Drawing for the job (mm, zero at the part's lowest x, y, z). A direction names the side the tool comes from. Give positions to 0.01 mm unless a question says otherwise; leave off trailing zeros. Order: outer loops, then holes, each group sorted by start corner. A loop starts at its lowest first (then second) coordinate and runs counter-clockwise, first axis right, second up. Notation, with made-up numbers: (23, 0) - (31, 0) arc R11 ccw to (31, 19) - close; hole circle Ø9 at (8, 51.5). An arc over 180 degrees is marked (long way). Use a Markdown table: item, result.
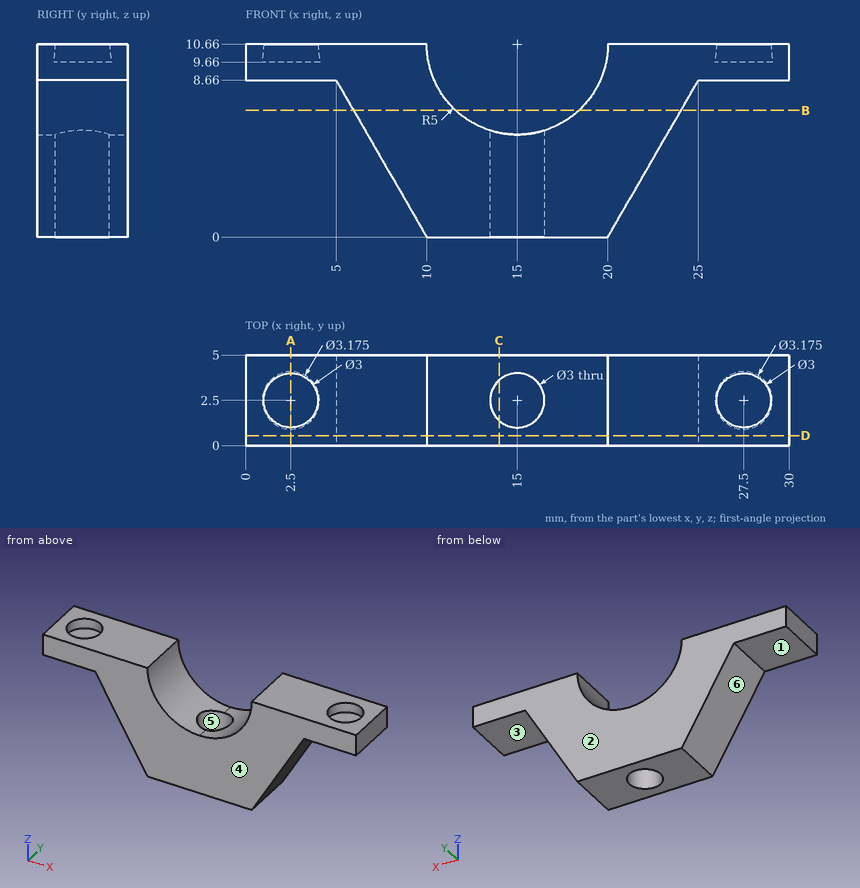
1) Two-plate mould, pull along X, no slides. Class the marked faces 4, 5 and 6: +X half, -X half, draft (parallel to the pull), parting line (faces both ways), or undercut.
Computed:
| item | result |
|---|---|
| face 4 | draft |
| face 5 | undercut |
| face 6 | -X half |
2) Slice it at D-D (y = 0.55). Write the cut outline in (x, z).
Computed:
| item | result |
|---|---|
| outline | (0, 8.66) - (5, 8.66) - (10, 0) - (20, 0) - (25, 8.66) - (30, 8.66) - (30, 10.66) - (20, 10.66) arc R5 cw to (10, 10.66) - (0, 10.66) - close |
3) Wall check: line 1 (Y direction, x = 15, z = 1.8); line 2 (Z direction, x = 27, y = 4.2); line 3 (X direction, y = 2.7, z = 5.75). Give the ranges that are in metal, low to high. Write a range as from..to.
Computed:
| item | result |
|---|---|
| line 1 | y = 0..1, 4..5 |
| line 2 | z = 8.66..10.66 |
| line 3 | x = 6.68..13.51, 16.49..23.32 |
4) Tool access for the marked faces 1, 2 and 3: list every direction of +Z, -Z, +X, -X, +Y, -Y with a clear straight run to the whole face (end or side of a thin tool).
Computed:
| item | result |
|---|---|
| face 1 | -Z, -X, +Y, -Y |
| face 2 | +Z, -Z, +X, -X, +Y |
| face 3 | -Z, +X, +Y, -Y |
5) Pin check, flat tip, straight feed: P1, Ø1.8, axis at x = 15, y = 2.5, coming from the +Z side. Stop position of the tip, or through.
Computed:
| item | result |
|---|---|
| P1 | passes through |
6) Slice it at B-B (z = 7). Write the cut outline in (x, y).
Computed:
| item | result |
|---|---|
| outline | (5.96, 0) - (11.59, 0) - (11.59, 5) - (5.96, 5) - close; (18.41, 0) - (24.04, 0) - (24.04, 5) - (18.41, 5) - close |
7) Slice it at A-A (x = 2.5). Write the cut outline in (y, z).
Computed:
| item | result |
|---|---|
| outline | (0, 8.66) - (5, 8.66) - (5, 10.66) - (4, 10.66) - (4.09, 9.66) - (0.91, 9.66) - (1, 10.66) - (0, 10.66) - close |
8) Slice it at C-C (x = 14). Write the cut outline in (y, z).
Computed:
| item | result |
|---|---|
| outline | (0, 0) - (1.38, 0) - (1.38, 5.76) - (0, 5.76) - close; (3.62, 0) - (5, 0) - (5, 5.76) - (3.62, 5.76) - close |
